```python
from build123d import *

# Parameters (mm, degrees)
SKETCH_1_W          = 65.796682854
SKETCH_1_H          = 7
EXTRUDE_1_DEPTH     = 1
SKETCH_1_3_W        = 65.796682854
SKETCH_1_3_H        = 7
EXTRUDE_4_DEPTH     = 1
SKETCH_2_R          = 1.6
SKETCH_2_W          = 15.527024866
SKETCH_2_H          = 4.354426868
EXTRUDE_5_DEPTH     = 10.2
SKETCH_3_W          = 11.091265895
SKETCH_3_H          = 1.250873396
EXTRUDE_6_DEPTH     = 8
EXTRUDE_7_DEPTH     = 8
SKETCH_5_R          = 1.55
CUT_EXTRUDE_1_DEPTH = 46.168181955
SKETCH_6_W          = 30.095890068
SKETCH_6_H          = 1.5
EXTRUDE_8_DEPTH     = 9
SKETCH_9_R          = 1.6
EXTRUDE_9_DEPTH     = 10.2
SKETCH_10_W         = 18.90463159
SKETCH_10_H         = 11.206527224
EXTRUDE_10_DEPTH    = 1.5
EXTRUDE_11_DEPTH    = 10
SKETCH_12_W         = 6.619618948
SKETCH_12_H         = 10.208127021
CUT_EXTRUDE_2_DEPTH = 4
SKETCH_13_W         = 5.420961308
SKETCH_13_H         = 7.723522143
EXTRUDE_12_DEPTH    = 8.7
SKETCH_14_R         = 1.6
CUT_EXTRUDE_3_DEPTH = 8
SKETCH_15_W         = 1.5
SKETCH_15_H         = 14.498100707
CUT_EXTRUDE_4_DEPTH = 9


with BuildPart() as part:
    # 草图1 → 凸台-拉伸1 (new body)
    with BuildSketch(Plane(origin=(0, 0, 0), x_dir=(1, 0, 0), z_dir=(0, 1, 0))):
        Polygon((21.783137071, 14), (-26.5, 14), (-26.5, 6.489174383), (-32.668192158, 6.489174383), (-32.668192158, 4.906407062), (-32.668192158, 3.5), (-31.253928934, 3.5), (-31.253928934, -3.5), (-32.668192158, -3.5), (-32.668192158, -4.906407062), (-32.668192158, -6.489174383), (-26.5, -6.489174383), (-26.5, -14), (21.783137071, -14), (23.783137071, -16), (23.783137071, -20.472436035), (25.783137071, -22.472436035), (44.687768661, -22.472436035), (44.687768661, -14), (44.687768661, 14), (44.687768661, 22.472436035), (39.670641652, 22.472436035), (39.670641652, 24.180906865), (37.700847745, 24.180906865), (25.783137071, 24.180906865), (23.783137071, 21.491786563), (23.783137071, 20.472436035), (23.783137071, 16), align=None)
        with Locations((4.125276897, 0)):
            Rectangle(SKETCH_1_W, SKETCH_1_H, mode=Mode.SUBTRACT)
    extrude(amount=EXTRUDE_1_DEPTH)

    # 草图1<3> → 凸台-拉伸4 (add)
    with BuildSketch(Plane(origin=(0, 0, 0), x_dir=(1, 0, 0), z_dir=(0, 1, 0))):
        Polygon((21.783137071, 14), (-26.5, 14), (-26.5, 6.489174383), (-32.668192158, 6.489174383), (-32.668192158, 4.906407062), (-32.668192158, 3.5), (-31.253928934, 3.5), (-31.253928934, -3.5), (-32.668192158, -3.5), (-32.668192158, -4.906407062), (-32.668192158, -6.489174383), (-26.5, -6.489174383), (-26.5, -14), (21.783137071, -14), (23.783137071, -16), (23.783137071, -20.472436035), (25.783137071, -22.472436035), (44.687768661, -22.472436035), (44.687768661, -14), (44.687768661, 14), (44.687768661, 22.472436035), (39.670641652, 22.472436035), (39.670641652, 24.180906865), (37.700847745, 24.180906865), (25.783137071, 24.180906865), (23.783137071, 21.491786563), (23.783137071, 20.472436035), (23.783137071, 16), align=None)
        with Locations((4.125276897, 0)):
            Rectangle(SKETCH_1_3_W, SKETCH_1_3_H, mode=Mode.SUBTRACT)
    extrude(amount=-EXTRUDE_4_DEPTH)

    # 草图2 → 凸台-拉伸5 (add)
    with BuildSketch(Plane(origin=(0, 1, 0), x_dir=(1, 0, 0), z_dir=(0, 1, 0))):
        with BuildLine():
            Line((32.873825551, -3.837422495), (20.961538439, -3.837422495))
            ThreePointArc((20.961538439, -3.837422495), (18.840218096, -4.716102152), (17.961538439, -6.837422495))
            Line((17.961538439, -6.837422495), (17.961538439, -9.071638955))
            Line((17.961538439, -9.071638955), (17.961538439, -13.050495751))
            Line((17.961538439, -13.050495751), (22.173089039, -13.050495751))
            Line((22.173089039, -13.050495751), (22.173089039, -9.071638955))
            Line((22.173089039, -9.071638955), (22.173089039, -5.615284864))
            Line((22.173089039, -5.615284864), (32.873825551, -5.615284864))
            Line((32.873825551, -5.615284864), (32.873825551, -3.837422495))
        make_face()
        with Locations((20.064403013, -9.071638955)):
            Circle(SKETCH_2_R, mode=Mode.SUBTRACT)
        Polygon((34.225317019, 6.570554911), (44.687768661, 6.570554911), (44.687768661, 11.265908811), (32.547793792, 11.265908811), (32.547793792, 4.534516494), (34.225317019, 4.534516494), align=None)
        with Locations((40.063673511, 8.987084634)):
            Circle(SKETCH_2_R, mode=Mode.SUBTRACT)
        with Locations((36.924256228, -20.295222601)):
            Rectangle(SKETCH_2_W, SKETCH_2_H)
        with Locations((40.063673511, -20.300345076)):
            Circle(SKETCH_2_R, mode=Mode.SUBTRACT)
    extrude(amount=EXTRUDE_5_DEPTH)

    # 草图3 → 凸台-拉伸6 (add)
    with BuildSketch(Plane.XZ.offset(1)):
        with Locations((-20.830181881, -13.374563302)):
            Rectangle(SKETCH_3_W, SKETCH_3_H)
        with Locations((-20.830181881, 13.374563302)):
            Rectangle(SKETCH_3_W, SKETCH_3_H)
    extrude(amount=-EXTRUDE_6_DEPTH)

    # 草图4 → 凸台-拉伸7 (add)
    with BuildSketch(Plane.XZ.offset(1)):
        Polygon((-14.752508247, -14), (-14.752508247, -19.024004183), (-16.715779154, -20.98727509), (-26.5, -20.98727509), (-26.5, -18.091791799), (-17.787107971, -18.091791799), (-17.787107971, -14), align=None)
        Polygon((-26.5, 20.98727509), (-26.5, 18.091791799), (-17.787107971, 18.091791799), (-17.787107971, 14), (-14.752508247, 14), (-14.752508247, 19.024004183), (-16.715779154, 20.98727509), align=None)
    extrude(amount=-EXTRUDE_7_DEPTH)

    # 草图5 → 切除-拉伸1 (cut, through all)
    with BuildSketch(Plane.XY.offset(20.98727509)):
        with Locations((-21.5, 4)):
            Circle(SKETCH_5_R)
    extrude(amount=-CUT_EXTRUDE_1_DEPTH, mode=Mode.SUBTRACT)

    # 草图6 → 凸台-拉伸8 (add)
    with BuildSketch(Plane(origin=(0, 1, 0), x_dir=(1, 0, 0), z_dir=(0, 1, 0))):
        with Locations((0.084132632, 4.25)):
            Rectangle(SKETCH_6_W, SKETCH_6_H)
        with Locations((0.084132632, -4.25)):
            Rectangle(SKETCH_6_W, SKETCH_6_H)
    extrude(amount=EXTRUDE_8_DEPTH)

    # 草图9 → 凸台-拉伸9 (add)
    with BuildSketch(Plane(origin=(0, 1, 0), x_dir=(1, 0, 0), z_dir=(0, 1, 0))):
        with BuildLine():
            Line((17.961538439, 6.837422495), (17.961538439, 13.050495751))
            Line((17.961538439, 13.050495751), (22.173089039, 13.050495751))
            Line((22.173089039, 13.050495751), (22.173089039, 5.615284864))
            Line((22.173089039, 5.615284864), (32.873825551, 5.615284864))
            Line((32.873825551, 5.615284864), (32.873825551, 3.837422495))
            Line((32.873825551, 3.837422495), (20.961538439, 3.837422495))
            ThreePointArc((20.961538439, 3.837422495), (18.840218096, 4.716102152), (17.961538439, 6.837422495))
        make_face()
        with Locations((20.064403013, 9.071638955)):
            Circle(SKETCH_9_R, mode=Mode.SUBTRACT)
    extrude(amount=EXTRUDE_9_DEPTH)

    # 草图10 → 凸台-拉伸10 (add)
    with BuildSketch(Plane(origin=(0, 1, 0), x_dir=(1, 0, 0), z_dir=(0, 1, 0))):
        with Locations((35.235452866, 16.869172423)):
            Rectangle(SKETCH_10_W, SKETCH_10_H)
    extrude(amount=EXTRUDE_10_DEPTH)

    # 草图11 → 凸台-拉伸11 (add)
    with BuildSketch(Plane.XZ.offset(1)):
        Polygon((32.547793792, -10.505295771), (25.467909356, -10.505295771), (25.467909356, -23.65934808), (38.4386145, -23.65934808), (38.4386145, -11.265908811), (40.863684521, -11.265908811), (40.863684521, -25.029182917), (24.636389842, -25.029182917), (21.547173342, -21.939966418), (20.550925149, -10.56366418), (24.129557088, -8.707277705), (32.547793792, -8.707277705), align=None)
    extrude(amount=-EXTRUDE_11_DEPTH)

    # 草图12 → 切除-拉伸2 (cut)
    with BuildSketch(Plane.XZ.offset(1)):
        with Locations((31.84517955, -17.496385448)):
            Rectangle(SKETCH_12_W, SKETCH_12_H)
    extrude(amount=-CUT_EXTRUDE_2_DEPTH, mode=Mode.SUBTRACT)

    # 草图13 → 凸台-拉伸12 (add)
    with BuildSketch(Plane(origin=(0, 2.5, 0), x_dir=(1, 0, 0), z_dir=(0, 1, 0))):
        with Locations((41.977288007, 18.610674964)):
            Rectangle(SKETCH_13_W, SKETCH_13_H)
    extrude(amount=EXTRUDE_12_DEPTH)

    # 草图14 → 切除-拉伸3 (cut)
    with BuildSketch(Plane(origin=(0, 11.2, 0), x_dir=(1, 0, 0), z_dir=(0, 1, 0))):
        with Locations((42.105027807, 19.921488723)):
            Circle(SKETCH_14_R)
    extrude(amount=-CUT_EXTRUDE_3_DEPTH, mode=Mode.SUBTRACT)

    # 草图15 → 切除-拉伸4 (cut, through all)
    with BuildSketch(Plane(origin=(0, 7, 0), x_dir=(1, 0, 0), z_dir=(0, 1, 0))):
        with Locations((-25.75, 13.738224737)):
            Rectangle(SKETCH_15_W, SKETCH_15_H)
        with Locations((-25.75, -13.738224737)):
            Rectangle(SKETCH_15_W, SKETCH_15_H)
    extrude(amount=-CUT_EXTRUDE_4_DEPTH, mode=Mode.SUBTRACT)


solid = part.part
```
Could you check a few things on this model? Use its own coordinates, in mm. A direction names the side the tool comes from. Coordinates: 2 decimals unless noted, no trailing zeros. Order: outer loops, then holes, each group sorted by start corner. A loop starts at its lowest first (then second) coordinate and runs counter-clockwise, first axis right, second up. Notation, with made-up numbers: M -31,69.25 L -13,69.25 A14 ccw -13,94.25 Z; hole C -32,-11.75 d5. An arc over 180 degrees is marked long. Use a Markdown table: item, result. Add a question column.
Q1. If I drill on L1, parallel to Y at x = -21.5, z = -19.35; L2, parallel to Z at x = 27, y = 10.75; L3, parallel to Z at x = 34, y = 0.5, over which ranges is the centre line in solid material (lowest first)?
Q2. Which directions (+Z, -Z, +X, -X, +Y, -Y) give clear straight access to the entire face, cutting with the end or side of a thin tool? Please do faces 5 (the cylindrical face through (18.795, 6.029, -8.098)), 6 (the flat face through (20, 6, 13.05)), 7 (the flat face through (29.161, 6, 20)), 8 (the flat face through (-25, 3, 20)), 9 (the flat face through (32.874, 6, 5)).
Q3. I want a section at A-A on x = -6. List the corners of the cut face in (y, z) for me.
Q4. I want a section at D-D on y = 4. Give the number of separate pieces and of enclosed holes in the cut face, then the cut area to 3 significant figures.
Q5. We'd pull the mould along X, two halves only. Please class faces 1 (the flat face through (35.155, 1, -18)), 2 (the flat face through (37, 2, -22.472)), 3 (the flat face through (39, 6, -6.571)), 4 (the flat face through (40.864, 6, -13)): pulls with the +X half, pulls with the -X half, needs draft (parallel to the pull), parting line crosses it, or undercut.
Q6. I want a section at C-C on x = 27. List the corners of the cut face in (y, z) for me, then the cut area to 3 significant figures.
Q7. I want a section at B-B on z = -16.5. List the corners of the cut face in (x, y) for me.
Q8. I'm going to push flat-ended pins straight in: pin 1 (0.8 mm diameter, centred on y = 5.5, z = -4.5, fed in from +X); pin 2 (1 mm diameter, centred on y = 5, z = 12, fed in from +X); pin 3 (1 mm diameter, centred on x = 31, z = 1.5, fed in from -Y); pin 4 (1.6 mm diameter, centred on x = -28.5, y = -0.5, fed in from -Z). Where does each tip first touch, or does it pass through?
Checked values:
| question | item | result |
|---|---|---|
| 1 | L1 | -1 to 2.45, 5.55 to 7 |
| 1 | L2 | -5.62 to -3.84, 3.84 to 5.62 |
| 1 | L3 | -25.03 to -22.6, -12.39 to -3.5, 3.5 to 22.47 |
| 2 | face 5 | +Y |
| 2 | face 6 | +Z, +X, +Y |
| 2 | face 7 | +Z, +Y |
| 2 | face 8 | +Z, -X, +Y, -Y |
| 2 | face 9 | +X, +Y |
| 3 | outline | M -1,-14 L 1,-14 L 1,-5 L 10,-5 L 10,-3.5 L -1,-3.5 Z; M -1,3.5 L 10,3.5 L 10,5 L 1,5 L 1,14 L -1,14 Z |
| 4 | separate pieces | 11 |
| 4 | enclosed holes | 7 |
| 4 | area | 521 mm² |
| 5 | face 1 | undercut |
| 5 | face 2 | undercut |
| 5 | face 3 | needs draft |
| 5 | face 4 | pulls with the +X half |
| 6 | outline | M -1,-25.03 L 9,-25.03 L 9,-23.66 L 1,-23.66 L 1,-22.47 L 2.5,-22.47 L 2.5,-11.27 L 1,-11.27 L 1,-10.51 L 9,-10.51 L 9,-8.71 L 1,-8.71 L 1,-5.62 L 11.2,-5.62 L 11.2,-3.84 L 1,-3.84 L 1,-3.5 L -1,-3.5 Z; M -1,3.5 L 1,3.5 L 1,3.84 L 11.2,3.84 L 11.2,5.62 L 1,5.62 L 1,22.47 L -1,22.47 Z |
| 6 | area | 159 mm² |
| 7 | outline | M -17.79,-1 L -14.75,-1 L -14.75,7 L -17.79,7 Z; M 21.07,-1 L 28.54,-1 L 28.54,2.5 L 25.78,2.5 L 25.78,1 L 25.47,1 L 25.47,9 L 21.07,9 Z; M 35.15,-1 L 44.69,-1 L 44.69,11.2 L 39.27,11.2 L 39.27,9 L 38.44,9 L 38.44,2.5 L 35.15,2.5 Z |
| 8 | pin 1 | x = 34.23 |
| 8 | pin 2 | x = 22.17 |
| 8 | pin 3 | through |
| 8 | pin 4 | z = -6.49 |
